Verification items for the finished model (mm, model axes). A direction names the side the tool comes from. Coordinates: 2 decimals unless noted, no trailing zeros. Loops run counter-clockwise (first coordinate to the right, second up) from the corner with the lowest first, then second, coordinate; pieces in that order, holes last. Notation, with made-up numbers: (45, -31.5) -> (50, -31.5) arc R10 ccw to (50, -21.5) -> close; hole circle Ø11 at (60.5, -2.5). An arc over 180 degrees is marked (long way). Use CSV: the item, a comma, the result in double quotes. Start each with the question number.
```python
from build123d import *

# Parameters (mm, degrees)
F1_DEPTH = 30
F3_DEPTH = 30
F4_R     = 2


with BuildPart() as f1:
    # F0 (on Top) → F1 (new body)
    with BuildSketch(Plane.XY):
        with BuildLine():
            Line((14.632652, 18.249727), (-44.452963, 14.977043))
            ThreePointArc((-44.452963, 14.977043), (-58.623402, 0), (-44.452963, -14.977043))
            Line((-44.452963, -14.977043), (14.632652, -18.249727))
            ThreePointArc((14.632652, -18.249727), (33.921183, 0), (14.632652, 18.249727))
        make_face()
    extrude(amount=F1_DEPTH)

    # F2 (on face) → F3 (cut)
    with BuildSketch(Plane.XY.offset(30)):
        with BuildLine():
            ThreePointArc((-43.899922, 4.992348), (-48.623402, 0), (-43.899922, -4.992348))
            Line((-43.899922, -4.992348), (15.185693, -8.265031))
            ThreePointArc((15.185693, -8.265031), (23.921183, 0), (15.185693, 8.265031))
            Line((15.185693, 8.265031), (-43.899922, 4.992348))
        make_face()
    extrude(amount=-F3_DEPTH, mode=Mode.SUBTRACT)

    # F4
    f4_edges = [f1.edges().sort_by_distance(p)[0] for p in [
        (-48.623402, 0, 30),
        (23.921183, 0, 30),
        (-14.357115, 6.62869, 30),
        (-14.910155, -16.613385, 30),
        (33.921183, 0, 30),
        (-14.910155, 16.613385, 30),
        (-58.623402, 0, 30),
        (-14.357115, -6.62869, 30),
    ]]
    fillet(f4_edges, radius=F4_R)


solid = f1.part
```
1. Set-up check for faces 4 (the flat face through (-14.497, 16.636, 13.804)), 5 (the cylindrical face through (-13.98, -7.25, 29.43)), 6 (the flat face through (-14.771, -6.606, 14.196)): record each of +Z, -Z, +X, -X, +Y, -Y from which the full face is reachable in a straight line by a thin tool's end or side.
2. Release check for a two-part mould opening along X. For faces 1 (the flat face through (-13, 11, 30)), 2 (the flat face through (-15.32, -16.59, 13.8)), 3 (the flat face through (-13.94, 6.65, 14.2)) record: released by +X, released by -X, zero draft, split by the parting line, or undercut.
3. Cross-section at A-A, the plane y = 0. Record the boundary of the cut face in (x, z), plus the area to 3 significant figures.
4. Depth check by flat-ended pin: pin 1 (6 mm diameter, centred on x = -49, z = 25.5, fed in from -Y); pin 2 (8 mm diameter, centred on x = 2.5, z = 11, fed in from -Y); pin 3 (3 mm diameter, centred on x = -22, z = 23.5, fed in from -Y). Enter the tip coordinate at first touch or a pass-through.
5. Cross-section at B-B, the plane z = 12. Record the boundary of the cut face in (x, y).
6. Scan lines: line 1 (Y direction, x = -8.5, z = 5); line 2 (Y direction, x = -21, z = 13); line 3 (X direction, y = 1, z = 17.5). Record each from-to range of solid material in increasing order.
Solution:
1,face 4,"+Z, -Z, -X, +Y"
1,face 5,"+Z"
1,face 6,"+Z, -Z"
2,face 1,"zero draft"
2,face 2,"released by -X"
2,face 3,"undercut"
3,outline,"(-58.62, 0) -> (-48.62, 0) -> (-48.62, 28) arc R2 ccw to (-50.62, 30) -> (-56.62, 30) arc R2 ccw to (-58.62, 28) -> close; (23.92, 0) -> (33.92, 0) -> (33.92, 28) arc R2 ccw to (31.92, 30) -> (25.92, 30) arc R2 ccw to (23.92, 28) -> close"
3,area,"597 mm2"
4,pin 1,"stops at y = -14.81"
4,pin 2,"stops at y = -17.8"
4,pin 3,"stops at y = -16.3"
5,outline,"(-44.45, -14.98) -> (14.63, -18.25) arc R18.28 ccw (long way) to (14.63, 18.25) -> (-44.45, 14.98) arc R15 ccw to start; hole (-43.9, -4.99) -> (15.19, -8.27) arc R8.28 ccw (long way) to (15.19, 8.27) -> (-43.9, 4.99) arc R5 ccw to start"
6,line 1,"y = -16.97 to -6.95, 6.95 to 16.97"
6,line 2,"y = -16.28 to -6.26, 6.26 to 16.28"
6,line 3,"x = -58.59 to -48.52, 23.86 to 33.89"
